Build history of the part. All positions in model axes, mm. A direction names the side the tool comes from. Round coordinates to 2 decimals unless told otherwise and drop trailing zeros. Write each loop counter-clockwise with the first axis right and the second up, starting at its lowest first coordinate (ties: lowest second). Pieces come first, ordered by that corner, then holes. Notation, with made-up numbers: (4, 38) - (56, 38) arc R28 cw to (56, 76) - close; hole circle Ø10 at (31.25, 85). An arc over 180 degrees is marked (long way). Answer as a JSON object with one key per item and string values. Group by question number.
Item 1: Two-plate mould, pull along Z, no slides. Class faces 1 (the cylindrical face through (-20.896, 0.07, -24.616)), 2 (the cylindrical face through (-17.8, 0.1, -11.7)), 3 (the flat face through (-19, -5, -3)), 4 (the cylindrical face through (11.73, 0.07, -17.28)): +Z half, -Z half, draft (parallel to the pull), parting line (faces both ways), or undercut.
Item 2: Which spindle directions (+Z, -Z, +X, -X, +Y, -Y) get a long thin tool onto all of the face, cutting with end or side? Do faces 5 (the flat face through (-29.4, -0.1, -15.984)), 6 (the flat face through (-19, 5, -3)), 7 (the cylindrical face through (10.4, 0.1, -15.3)), 8 (the cylindrical face through (-28.266, 0.07, -15.733)), 9 (the cylindrical face through (-32.814, 0.07, 6.622)). Say none if no direction does.
Item 3: Slice it at C-C, the plane z = 0. List the corners of the cut face in (x, y), then the cut area to 3 significant figures.
Item 4: Slice it at A-A, the plane x = 0. List the corners of the cut face in (y, z).
Item 5: Slice it at D-D, the plane z = 12. List the corners of the cut face in (x, y).
Item 6: Flat gauge pins, fed straight in: pin 1 (1 mm diameter, centred on y = 4, z = 5, fed in from +X); pin 2 (19 mm diameter, centred on x = -22, z = -15.98, fed in from -Y); pin 3 (3 mm diameter, centred on y = 0, z = -20, fed in from -X); pin 4 (2 mm diameter, centred on x = -24.5, y = -1.5, fed in from -Z). Where does each tip first touch, or does it go through?
Item 7: Probe line 1 (Z direction, x = 0, y = 2.5); line 2 (Z direction, x = -2, y = 3); line 3 (X direction, y = -2, z = 0). List the from-to ranges inside material, lowest first. Write a range as from..to.
Item 8: Slice it at B-B, the plane z = -13.5. List the corners of the cut face in (x, y).
from build123d import *

# Parameters (mm, degrees)
F0_R     = 6
F1_DEPTH = 5
F2_R     = 2
F3_COUNT = 2
F3_ANGLE = 36
F5_DEPTH = 10.0010001
F6_R     = 1


with BuildPart() as f1:
    # F0 (on Front) → F1 (new body, symmetric)
    with BuildSketch(Plane.XZ):
        with BuildLine():
            ThreePointArc((-20.3662859317, 5.8640119715), (-18.7542946844, 3.1267729293), (-18.1936839424, 0))
            ThreePointArc((-18.1936839424, 0), (-18.7542946844, -3.1267729293), (-20.3662859317, -5.8640119715))
            ThreePointArc((-20.3662859317, -5.8640119715), (2.9610481198, -20.9858150446), (21.1936839424, 0))
            ThreePointArc((21.1936839424, 0), (2.9610481198, 20.9858150446), (-20.3662859317, 5.8640119715))
        make_face()
        with BuildLine():
            ThreePointArc((-18.1936839424, 0), (0, 18.1936839424), (18.1936839424, 0))
            ThreePointArc((18.1936839424, 0), (0, -18.1936839424), (-18.1936839424, 0))
        make_face(mode=Mode.SUBTRACT)
        with BuildLine():
            ThreePointArc((-20.3662859317, -5.8640119715), (-18.7542946844, -3.1267729293), (-18.1936839424, 0))
            ThreePointArc((-18.1936839424, 0), (-18.7542946844, 3.1267729293), (-20.3662859317, 5.8640119715))
            ThreePointArc((-20.3662859317, 5.8640119715), (-20.9858150446, 2.9610481198), (-21.1936839424, 0))
            ThreePointArc((-21.1936839424, 0), (-20.9858150446, -2.9610481198), (-20.3662859317, -5.8640119715))
        make_face()
        with BuildLine():
            ThreePointArc((-21.1936839424, 0), (-20.9858150446, 2.9610481198), (-20.3662859317, 5.8640119715))
            ThreePointArc((-20.3662859317, 5.8640119715), (-36.1936839424, 0), (-20.3662859317, -5.8640119715))
            ThreePointArc((-20.3662859317, -5.8640119715), (-20.9858150446, -2.9610481198), (-21.1936839424, 0))
        make_face()
        with Locations((-27.1936839424, 0)):
            Circle(F0_R, mode=Mode.SUBTRACT)
    extrude(amount=F1_DEPTH, both=True)

    # F2
    f2_edges = [f1.edges().sort_by_distance(p)[0] for p in [
        (-20.366286, 0, 5.864012),
        (-20.366286, 0, -5.864012),
    ]]
    fillet(f2_edges, radius=F2_R)

    # F3: F1 ×2 about axis
    f3_axis = Axis((0, 0, 0), (0, -1, 0))


with BuildPart() as f1_1:
    add(f1.part)
    for i in range(1, F3_COUNT):
        add(f1.part.rotate(f3_axis, i * F3_ANGLE / (F3_COUNT - 1)))

    # F4 (on face) → F5 (cut, through all)
    with BuildSketch(Plane.XZ.offset(5)):
        with BuildLine():
            ThreePointArc((-31.2472251881, -4.4236640209), (-33.1936839424, 0), (-31.2472251881, 4.4236640209))
            Line((-31.2472251881, 4.4236640209), (-33.273995811, 6.6354960313))
            ThreePointArc((-33.273995811, 6.6354960313), (-36.1936839424, 0), (-33.273995811, -6.6354960313))
            Line((-33.273995811, -6.6354960313), (-31.2472251881, -4.4236640209))
        make_face()
        with BuildLine():
            ThreePointArc((12.1561977089, -17.3608495275), (21.1936839424, 0), (12.1561977089, 17.3608495275))
            Line((12.1561977089, 17.3608495275), (10.4354683998, 14.9033933946))
            ThreePointArc((10.4354683998, 14.9033933946), (16.1379947524, 8.4009083301), (18.1936839424, 0))
            ThreePointArc((18.1936839424, 0), (16.1379947524, -8.4009083301), (10.4354683998, -14.9033933946))
            Line((10.4354683998, -14.9033933946), (12.1561977089, -17.3608495275))
        make_face()
        with BuildLine():
            Line((-28.0001524491, -15.9840463769), (-31.0001524491, -15.9840463769))
            ThreePointArc((-31.0001524491, -15.9840463769), (-28.0804643176, -22.6195424082), (-21.2157507644, -24.9497986597))
            Line((-21.2157507644, -24.9497986597), (-21.4772179926, -21.9612145654))
            ThreePointArc((-21.4772179926, -21.9612145654), (-26.0536936948, -20.4077103977), (-28.0001524491, -15.9840463769))
        make_face()
    extrude(amount=-F5_DEPTH, mode=Mode.SUBTRACT)

    # F6
    f6_edges = [f1_1.edges().sort_by_distance(p)[0] for p in [
        (-31.247225, 0, 4.423664),
        (-33.273996, 0, 6.635496),
        (-33.273996, 0, -6.635496),
        (-31.247225, 0, -4.423664),
        (10.435468, 0, 14.903393),
        (12.156198, 0, 17.36085),
        (12.156198, 0, -17.36085),
        (10.435468, 0, -14.903393),
        (-28.000152, 0, -15.984046),
        (-31.000152, 0, -15.984046),
        (-21.477218, 0, -21.961215),
        (-21.215751, 0, -24.949799),
    ]]
    fillet(f6_edges, radius=F6_R)


solid = f1_1.part
Geometry says:
{
 "1": {"face 1": "-Z half", "face 2": "undercut", "face 3": "draft", "face 4": "undercut"},
 "2": {"face 5": "-Z, -X, +Y, -Y", "face 6": "+Z, -Z, +X, -X, +Y", "face 7": "+Y, -Y", "face 8": "-Z, +Y, -Y", "face 9": "-X, +Y, -Y"},
 "3": {"outline": "(-21.19, -5) - (-18.19, -5) - (-18.19, 5) - (-21.19, 5) - close", "area": "30.0 mm^2"},
 "4": {"outline": "(-5, -21.19) - (5, -21.19) - (5, -18.19) - (-5, -18.19) - close; (-5, 18.19) - (5, 18.19) - (5, 21.19) - (-5, 21.19) - close"},
 "5": {"outline": "(-17.47, -5) - (-13.68, -5) - (-13.68, 5) - (-17.47, 5) - close"},
 "6": {"pin 1": "stops at x = -17.34", "pin 2": "stops at y = -5", "pin 3": "stops at x = -19.64", "pin 4": "stops at z = -11.11"},
 "7": {"line 1": "z = -21.19..-18.19, 18.19..21.19", "line 2": "z = -21.1..-18.08, 18.08..21.1", "line 3": "x = -21.19..-18.19"},
 "8": {"outline": "(-30.65, -5) - (-27.46, -5) - (-27.46, 5) - (-30.65, 5) - close; (-16.54, -5) - (-12.2, -5) - (-12.2, 5) - (-16.54, 5) - close"}
}
